Source: three-view drawing plus pictorial views. Frame: mm from the lowest corner of the part. A direction names the side the tool comes from. Give positions to 0.01 mm unless a question says otherwise; leave off trailing zeros. Loops run counter-clockwise (first coordinate to the right, second up) from the corner with the lowest first, then second, coordinate; pieces in that order, holes last. Notation, with made-up numbers: M -35,14 L 8,14 A19 ccw 8,22 Z; hole C 0,-31.75 d7. An arc over 180 degrees is marked long. Write item = value, one per line.
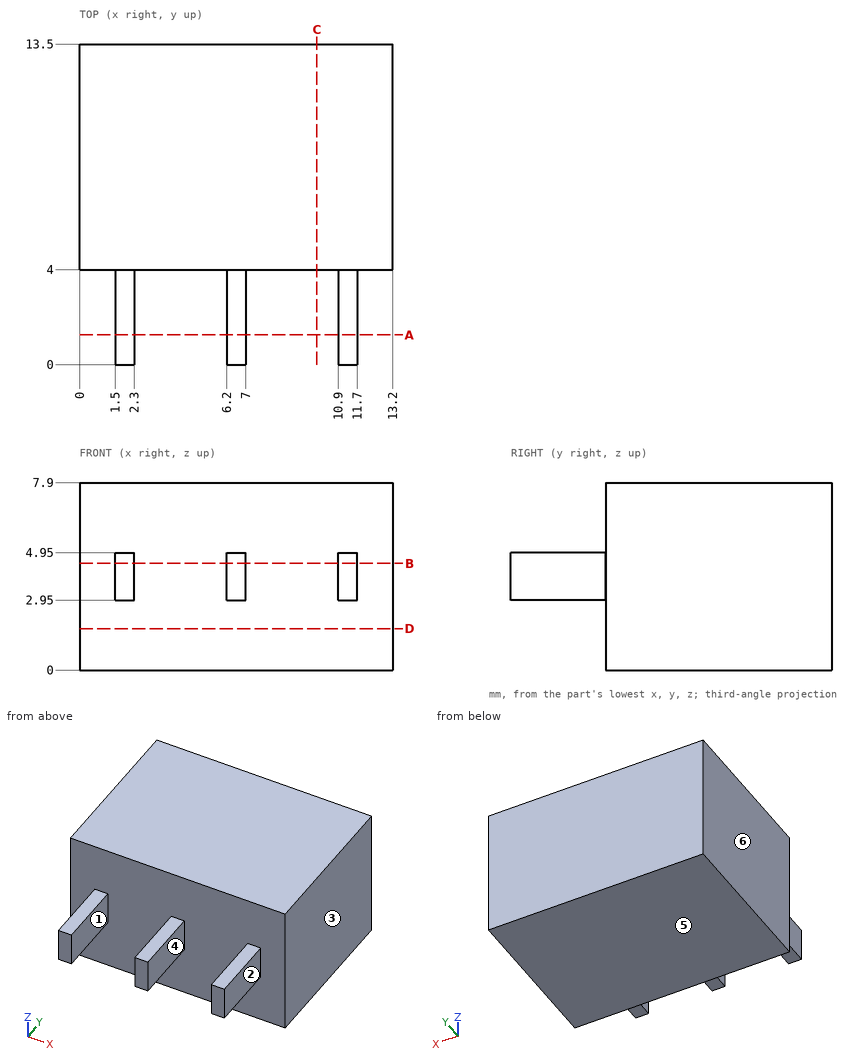
1. Reachability of the marked faces 1, 2 and 3 from +Z, -Z, +X, -X, +Y, -Y: full face, straight path, thin tool, end or side. Return the list, or none.
Derived:
face_1 = +Z, -Z, -Y
face_2 = +Z, -Z, +X, -Y
face_3 = +Z, -Z, +X, +Y, -Y
2. First-contact query: pin 1 Ø0.6 at (y, z) = (2, 4.5) entering from +X; pin 2 Ø2 at (y, z) = (2.5, 3.5) entering from -X; pin 3 Ø0.9 at (x, y) = (6.5, 1) entering from +Z. Flat tips, straight axial feed; report the tip coordinate or a pass-through.
Derived:
pin_1 = 11.7
pin_2 = 1.5
pin_3 = 4.95
3. Cut plane B-B, the plane z = 4.5. Return the cut outline in (x, y).
Derived:
outline = M 0,4 L 1.5,4 L 1.5,0 L 2.3,0 L 2.3,4 L 6.2,4 L 6.2,0 L 7,0 L 7,4 L 10.9,4 L 10.9,0 L 11.7,0 L 11.7,4 L 13.2,4 L 13.2,13.5 L 0,13.5 Z
4. Pull-direction query (X, two-part tool) for the marked faces 4, 5 and 6; classes: +X half, -X half, draft (parallel to the pull), parting line (faces both ways), or undercut.
Derived:
face_4 = undercut
face_5 = draft
face_6 = -X half
5. Cut plane D-D, the plane z = 1.75. Return the cut outline in (x, y).
Derived:
outline = M 0,4 L 13.2,4 L 13.2,13.5 L 0,13.5 Z
6. Material intervals for probe 1 along X at (y, z) = (2.75, 3.25); probe 2 along Y at (x, z) = (3.5, 5.25), sorted ascending. Write a range as from..to.
Derived:
probe_1 = 1.5..2.3, 6.2..7, 10.9..11.7
probe_2 = 4..13.5
7. Cut plane C-C, the plane x = 10. Return the cut outline in (y, z), then the cut area to 4 significant figures.
Derived:
outline = M 4,0 L 13.5,0 L 13.5,7.9 L 4,7.9 Z
area = 75.05 mm²
8. Cut plane A-A, the plane y = 1.25. Return the cut outline in (x, z), then the cut area to 3 significant figures.
Derived:
outline = M 1.5,2.95 L 2.3,2.95 L 2.3,4.95 L 1.5,4.95 Z; M 6.2,2.95 L 7,2.95 L 7,4.95 L 6.2,4.95 Z; M 10.9,2.95 L 11.7,2.95 L 11.7,4.95 L 10.9,4.95 Z
area = 4.80 mm²
